CAD build for the part. Positions are in the model's coordinates, mm. Face numbers are marked on the shaded views. A direction names the side the tool comes from. Give positions to 0.01 mm unless a question says otherwise; leave off trailing zeros. Write each loop counter-clockwise with the first axis right and the second up, starting at its lowest first coordinate (ties: lowest second). Pieces come first, ordered by that corner, then holes. Notation, with made-up numbers: (85, 20.25) - (129, 20.25) arc R13 cw to (129, 35.25) - close; hole circle Ø7 at (-31.5, 9). An arc over 180 degrees is marked (long way). Put each result on its own line as item: value. Start each with the question number.
1. Cut at C-C on z = 9. List the corners of the cut face in (x, y).
2. Cut at A-A on y = 34.5. List the corners of the cut face in (x, z), and give its area (3 significant figures).
3. Tool access for the marked faces 1, 2 and 3: list every direction of +Z, -Z, +X, -X, +Y, -Y with a clear straight run to the whole face (end or side of a thin tool).
4. Wall check: line 1 (Z direction, x = -15.5, y = 36.65); line 2 (X direction, y = 35, z = 15). Give the ranges that are in metal, low to high.
5. Cut at B-B on x = 5. List the corners of the cut face in (y, z).
6. Drop flat-ended pins along their axis: pin 1 (1 mm diameter, centred on x = -3.5, z = 0, fed in from +Y); pin 2 (1.5 mm diameter, centred on x = -13.5, z = -19.5, fed in from -Y); pin 3 (5.5 mm diameter, centred on y = 3.5, z = -24, fed in from -X); pin 4 (9.5 mm diameter, centred on x = -3, y = 25.5, fed in from -Z). Give the stop position or say it passes through.
7. Mould opens along Y. For the marked faces 4, 5 and 6 say: +Y half, -Y half, draft (parallel to the pull), parting line (faces both ways), or undercut.
8. Cut at D-D on y = 41. List the corners of the cut face in (x, z), and give its area (3 significant figures).
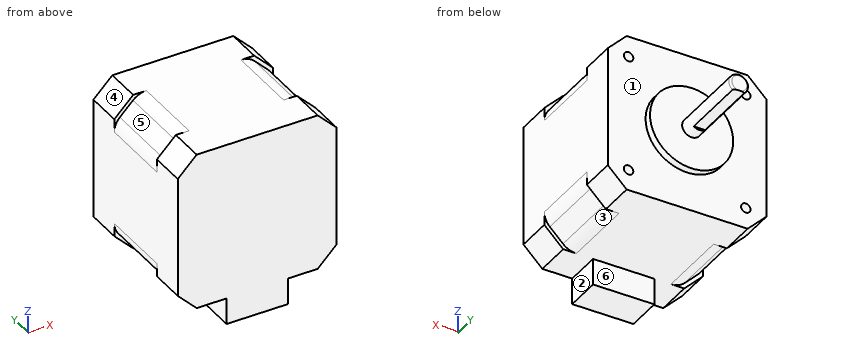
from build123d import *

# Parameters (mm, degrees)
SKETCH1_W             = 42
SKETCH1_H             = 42
BOSS_EXTRUDE1_DEPTH   = 38
SKETCH2_R             = 11
BOSS_EXTRUDE2_DEPTH   = 2
SKETCH3_R             = 2.5
BOSS_EXTRUDE3_DEPTH   = 3.5
BOSS_EXTRUDE4_DEPTH   = 18
M3_TAPPED_HOLE1_D     = 2.5
M3_TAPPED_HOLE1_DEPTH = 5
M3_TAPPED_HOLE1_TIP   = 0.751075774
CHAMFER1_SIZE         = 5
SKETCH11_W            = 10
SKETCH11_H            = 19.2
CUT_EXTRUDE2_DEPTH    = 1
SKETCH12_W            = 10
SKETCH12_H            = 19.2
CUT_EXTRUDE3_DEPTH    = 1
SKETCH13_W            = 10
SKETCH13_H            = 19.2
CUT_EXTRUDE4_DEPTH    = 1
SKETCH14_W            = 10
SKETCH14_H            = 19.2
CUT_EXTRUDE5_DEPTH    = 1
FILLET1_R             = 5
SKETCH15_W            = 16.2
SKETCH15_H            = 9.4
BOSS_EXTRUDE5_DEPTH   = 7
FILLET3_R             = 0.5


with BuildPart() as part:
    # Sketch1 → Boss-Extrude1 (new body)
    with BuildSketch(Plane(origin=(0, 0, 0), x_dir=(1, 0, 0), z_dir=(0, 1, 0))):
        Rectangle(SKETCH1_W, SKETCH1_H)
    extrude(amount=BOSS_EXTRUDE1_DEPTH)

    # Sketch2 → Boss-Extrude2 (add)
    with BuildSketch(Plane(origin=(0, 38, 0), x_dir=(1, 0, 0), z_dir=(0, 1, 0))):
        with Locations(Location((0, 0, 0), (0, 0, 270))):
            Circle(SKETCH2_R)
    extrude(amount=BOSS_EXTRUDE2_DEPTH)

    # Sketch3 → Boss-Extrude3 (add)
    with BuildSketch(Plane(origin=(0, 40, 0), x_dir=(1, 0, 0), z_dir=(0, 1, 0))):
        with Locations(Location((0, 0, 0), (0, 0, 270))):
            Circle(SKETCH3_R)
    extrude(amount=BOSS_EXTRUDE3_DEPTH)

    # Sketch4 → Boss-Extrude4 (add)
    with BuildSketch(Plane(origin=(0, 43.5, 0), x_dir=(1, 0, 0), z_dir=(0, 1, 0))):
        with BuildLine():
            ThreePointArc((-1.5, 2), (-2.371708245, -0.790569415), (0, -2.5))
            Line((0, -2.5), (0, 2))
            Line((0, 2), (-1.5, 2))
        make_face()
        with BuildLine():
            Line((0, 2), (0, -2.5))
            ThreePointArc((0, -2.5), (1.767766953, -1.767766953), (2.5, 0))
            ThreePointArc((2.5, 0), (2.236067977, 1.118033989), (1.5, 2))
            Line((1.5, 2), (0, 2))
        make_face()
    extrude(amount=BOSS_EXTRUDE4_DEPTH)

    # M3 Tapped Hole1
    with Locations(Plane(origin=(0, 38, 0), x_dir=(1, 0, 0), z_dir=(0, 1, 0))):
        with Locations((-15.5, 15.5), (15.5, 15.5), (15.5, -15.5), (-15.5, -15.5)):
            Hole(M3_TAPPED_HOLE1_D / 2, depth=M3_TAPPED_HOLE1_DEPTH)
            with Locations((0, 0, -(M3_TAPPED_HOLE1_DEPTH + M3_TAPPED_HOLE1_TIP / 2))):  # 118° drill point
                Cone(0, M3_TAPPED_HOLE1_D / 2, M3_TAPPED_HOLE1_TIP, mode=Mode.SUBTRACT)

    # Chamfer1
    chamfer1_edges = [part.edges().sort_by_distance(p)[0] for p in [
        (-21, 19, -21),
        (21, 19, -21),
        (21, 19, 21),
        (-21, 19, 21),
    ]]
    chamfer(chamfer1_edges, length=CHAMFER1_SIZE)

    # Sketch11 → Cut-Extrude2 (cut)
    with BuildSketch(Plane(origin=(18.5, 0, 18.5), x_dir=(0.7071067811865485, 0, -0.7071067811865467), z_dir=(0.7071067811865467, 0, 0.7071067811865485))):
        with Locations((0, 19)):
            Rectangle(SKETCH11_W, SKETCH11_H)
    extrude(amount=-CUT_EXTRUDE2_DEPTH, mode=Mode.SUBTRACT)

    # Sketch12 → Cut-Extrude3 (cut)
    with BuildSketch(Plane(origin=(-18.5, 0, 18.5), x_dir=(0.7071067811865465, 0, 0.7071067811865487), z_dir=(-0.7071067811865487, 0, 0.7071067811865465))):
        with Locations((0, 19)):
            Rectangle(SKETCH12_W, SKETCH12_H)
    extrude(amount=-CUT_EXTRUDE3_DEPTH, mode=Mode.SUBTRACT)

    # Sketch13 → Cut-Extrude4 (cut)
    with BuildSketch(Plane(origin=(-18.5, 0, -18.5), x_dir=(-0.7071067811865485, 0, 0.7071067811865467), z_dir=(-0.7071067811865467, 0, -0.7071067811865485))):
        with Locations((0, 19)):
            Rectangle(SKETCH13_W, SKETCH13_H)
    extrude(amount=-CUT_EXTRUDE4_DEPTH, mode=Mode.SUBTRACT)

    # Sketch14 → Cut-Extrude5 (cut)
    with BuildSketch(Plane(origin=(18.5, 0, -18.5), x_dir=(-0.7071067811865467, 0, -0.7071067811865485), z_dir=(0.7071067811865485, 0, -0.7071067811865467))):
        with Locations((0, 19)):
            Rectangle(SKETCH14_W, SKETCH14_H)
    extrude(amount=-CUT_EXTRUDE5_DEPTH, mode=Mode.SUBTRACT)

    # Fillet1
    fillet1_edges = [part.edges().sort_by_distance(p)[0] for p in [
        (-14.585786438, 19, 21),
        (-21, 19, 14.585786438),
        (-14.585786438, 19, -21),
        (-21, 19, -14.585786438),
        (14.585786438, 19, -21),
        (21, 19, -14.585786438),
        (21, 19, 14.585786438),
        (14.585786438, 19, 21),
    ]]
    fillet(fillet1_edges, radius=FILLET1_R)

    # Sketch15 → Boss-Extrude5 (add)
    with BuildSketch(Plane(origin=(0, 0, -21), x_dir=(-1, 0, 0), z_dir=(0, 0, -1))):
        with Locations((0, 4.7)):
            Rectangle(SKETCH15_W, SKETCH15_H)
    extrude(amount=BOSS_EXTRUDE5_DEPTH)

    # Fillet3
    # the kernel refuses this fillet: 0.5 mm, written as the material it takes off along each edge
    with BuildSketch(Plane(origin=(0, 61.5, 0), x_dir=(0.14099255813885567, 0, -0.990010655775715), z_dir=(-0.990010655775715, 0, -0.14099255813885567))) as fillet3_piece_1:
        with BuildLine():
            CenterArc((2.5 - FILLET3_R, FILLET3_R), FILLET3_R, 270, 90)
            Line((2.5 - FILLET3_R, 0), (2.5, 0))
            Line((2.5, 0), (2.5, FILLET3_R))
        make_face()
    revolve(axis=Axis((0, 61.5, 0), (0, -1, 0)), revolution_arc=343.789429262, mode=Mode.SUBTRACT)


solid = part.part
Report:
1. outline: (-21, 0) - (21, 0) - (21, 38) - (6.32, 38) - (6.32, 40) - (-6.32, 40) - (-6.32, 38) - (-21, 38) - close
2. outline: (-21, -16) - (-16, -21) - (16, -21) - (21, -16) - (21, 16) - (16, 21) - (-16, 21) - (-21, 16) - close; hole circle Ø2.5 at (-15.5, -15.5); hole circle Ø2.5 at (-15.5, 15.5); hole circle Ø2.5 at (15.5, -15.5); hole circle Ø2.5 at (15.5, 15.5)
2. area: 1,690 mm²
3. face 1: +Y
3. face 2: -Z, +X, +Y, -Y
3. face 3: -Z, +X
4. line 1: z = -21 to -16.75, -14.25 to 14.25, 16.75 to 21
4. line 2: x = -21 to -16.65, -14.35 to 14.35, 16.65 to 21
5. outline: (0, -28) - (9.4, -28) - (9.4, -21) - (38, -21) - (38, -9.8) - (40, -9.8) - (40, 9.8) - (38, 9.8) - (38, 21) - (0, 21) - close
6. pin 1: stops at y = 40
6. pin 2: stops at y = 0
6. pin 3: stops at x = -8.1
6. pin 4: stops at z = -21
7. face 4: draft
7. face 5: undercut
7. face 6: +Y half
8. outline: circle Ø5 at (0, 0)
8. area: 19.6 mm²
